```python
from build123d import *

# Parameters (mm, degrees)
ESBO_O1_R                = 17.25
ESBO_O1_R_2              = 4.5
RESSALTO_EXTRUS_O1_DEPTH = 20
CORTE_EXTRUS_O1_DEPTH    = 8
ESBO_O5_R                = 2.75
ESBO_O5_R_2              = 1.75
RESSALTO_EXTRUS_O2_DEPTH = 5.5
FILETE1_R                = 5
FILETE2_R                = 10
ESBO_O7_R                = 6.5
ESBO_O7_R_2              = 4.5
RESSALTO_EXTRUS_O3_DEPTH = 7
FILETE3_R                = 5
CHANFRO1_SIZE            = 1


with BuildPart() as part:
    # Esboço1 → Ressalto-extrusão1 (new body)
    with BuildSketch(Plane(origin=(0, 0, 0), x_dir=(1, 0, 0), z_dir=(0, 1, 0))):
        with Locations(Location((0, 0, 0), (0, 0, 270))):
            Circle(ESBO_O1_R)
        with Locations(Location((0, 0, 0), (0, 0, 270))):
            Circle(ESBO_O1_R_2, mode=Mode.SUBTRACT)
    extrude(amount=RESSALTO_EXTRUS_O1_DEPTH)

    # Esboço1<3> → Corte-extrusão1 (cut)
    with BuildSketch(Plane(origin=(0, 0, 0), x_dir=(1, 0, 0), z_dir=(0, 1, 0))):
        Polygon((-6.75, 3.897114317), (-6.75, -3.897114317), (0, -7.794228634), (6.75, -3.897114317), (6.75, 3.897114317), (0, 7.794228634), align=None)
    extrude(amount=CORTE_EXTRUS_O1_DEPTH, mode=Mode.SUBTRACT)

    # Esboço5 → Ressalto-extrusão2 (add)
    # profile 1 of 2: a face of its own
    with BuildSketch(Plane.XZ):
        with BuildLine():
            Line((-17.25, 10), (-14.055692797, 10))
            ThreePointArc((-14.055692797, 10), (-17.25, 0), (-14.055692797, -10))
            Line((-14.055692797, -10), (-17.25, -10))
            Line((-17.25, -10), (-37.25, -10))
            Line((-37.25, -10), (-37.25, 10))
            Line((-37.25, 10), (-17.25, 10))
        make_face()
        with Locations(Location((-27.25, 0, 0), (0, 0, 270))):
            Circle(ESBO_O5_R, mode=Mode.SUBTRACT)
    # profile 2 of 2: a face of its own
    with BuildSketch(Plane.XZ):
        with BuildLine():
            Line((-10, 17.25), (-10, 14.055692797))
            ThreePointArc((-10, 14.055692797), (0, 17.25), (10, 14.055692797))
            Line((10, 14.055692797), (10, 17.25))
            Line((10, 17.25), (10, 37.25))
            Line((10, 37.25), (-10, 37.25))
            Line((-10, 37.25), (-10, 17.25))
        make_face()
        with Locations(Location((0, 27.25, 0), (0, 0, 270))):
            Circle(ESBO_O5_R_2, mode=Mode.SUBTRACT)
    extrude(amount=-RESSALTO_EXTRUS_O2_DEPTH)

    # Filete1
    filete1_edges = [part.edges().sort_by_distance(p)[0] for p in [
        (-14.055692797, 2.75, -10),
        (-17.25, 5.5, 0),
        (-14.055692797, 2.75, 10),
        (-5.248895086, 5.5, 16.432029709),
        (10, 2.75, 14.055692797),
        (-10, 2.75, 14.055692797),
    ]]
    fillet(filete1_edges, radius=FILETE1_R)

    # Filete2
    filete2_edges = [part.edges().sort_by_distance(p)[0] for p in [
        (10, 2.75, 37.25),
        (-10, 2.75, 37.25),
        (-37.25, 2.75, -10),
        (-37.25, 2.75, 10),
    ]]
    fillet(filete2_edges, radius=FILETE2_R - 0.0001)  # a hair under: the kernel refuses the full size

    # Esboço7 → Ressalto-extrusão3 (add)
    with BuildSketch(Plane(origin=(0, 20, 0), x_dir=(1, 0, 0), z_dir=(0, 1, 0))):
        with Locations(Location((0, 0, 0), (0, 0, 270))):
            Circle(ESBO_O7_R)
        with Locations(Location((0, 0, 0), (0, 0, 270))):
            Circle(ESBO_O7_R_2, mode=Mode.SUBTRACT)
    extrude(amount=RESSALTO_EXTRUS_O3_DEPTH)

    # Filete3
    filete3_edges = [part.edges().sort_by_distance(p)[0] for p in [
        (0, 20, -6.5),
    ]]
    fillet(filete3_edges, radius=FILETE3_R)

    # Chanfro1
    chanfro1_edges = [part.edges().sort_by_distance(p)[0] for p in [
        (0, 27, -6.5),
    ]]
    chamfer(chanfro1_edges, length=CHANFRO1_SIZE)


solid = part.part
```
CAD build for the part. Positions are in the model's coordinates, mm. A direction names the side the tool comes from. Round coordinates to 2 decimals unless told otherwise and drop trailing zeros. Order: outer loops, then holes, each group sorted by start corner. A loop starts at its lowest first (then second) coordinate and runs counter-clockwise, first axis right, second up.
Item 1: Mould opens along X. For faces 1 (the face through (-10, 3, 22)), 2 (the face through (-24.523, 2.712, 0.358)), 3 (the face through (0, 27, -5)) say: pulls with the +X half, pulls with the -X half, needs draft (parallel to the pull), parting line crosses it, or undercut.
Item 2: Saw through at A-A on x = -33. Write the cut outline in (y, z).
Item 3: Pin check, flat tips, straight feed: pin 1 (3 mm diameter, centred on y = 16, z = -10, fed in from -X); pin 2 (12 mm diameter, centred on x = -20, y = 3.5, fed in from -Z); pin 3 (5 mm diameter, centred on x = -7.5, y = 5, fed in from +Z). Stop position of each tip, or through.
Item 4: Saw through at B-B on z = 30. Write the cut outline in (x, y).
Item 5: Tool access for faces 4 (the face through (11.66, 12.08, -12.71)), 5 (the face through (-3.33, 3.94, -5.87)), 6 (the face through (-22, 3, -10)): list every direction of +Z, -Z, +X, -X, +Y, -Y with a clear straight run to the whole face (end or side of a thin tool).
Item 6: Probe line 1 along X through (y, z) = (3.9, 27.25); line 2 along X through (y, z) = (16.5, 0). List the from-to ranges inside material, lowest first.
Reported:
1. face 1: pulls with the -X half
1. face 2: undercut
1. face 3: needs draft
2. outline: (0, -8.18) - (5.5, -8.18) - (5.5, 8.18) - (0, 8.18) - close
3. pin 1: stops at x = -15.01
3. pin 2: stops at z = -10.63
3. pin 3: stops at z = 35.91
4. outline: (-9.61, 0) - (9.61, 0) - (9.61, 5.5) - (-9.61, 5.5) - close
5. face 4: +Y
5. face 5: -Y
5. face 6: -Z, -X, +Y, -Y
6. line 1: x = -10 to -1.75, 1.75 to 10
6. line 2: x = -17.25 to -4.5, 4.5 to 17.25
